Part model, mm, in its own coordinate system. A direction names the side the tool comes from. Coordinates: 2 decimals unless noted, no trailing zeros. Loops run counter-clockwise (first coordinate to the right, second up) from the corner with the lowest first, then second, coordinate; pieces in that order, holes last. Notation, with made-up numbers: (53.5, 66) -> (96.5, 66) arc R12 cw to (96.5, 89) -> close; hole circle Ø8 at (63.5, -3.5). An arc over 180 degrees is marked (long way). Use one line per item in the form item = value. Start each with the question number.
(1) Drill centre lines: L1, parallel to Z at x = 8, y = 1.5; L2, parallel to Z at x = 0.95, y = 17; L3, parallel to X at y = 23, z = 14.5. Where is each one in solid material? Low to high. Write a range as [from, to].
(2) Pin check, flat tips, straight feed: P1, Ø1.5, axis at x = 7, z = 2.5, coming from the +Y side; P2, Ø12.5, axis at y = 15, z = 15.5, coming from the +X side. Stop position of each tip, or through.
(3) Band-saw the part on A-A on z = 12.5. Give the cut face in (x, y), then the cut area to 3 significant figures.
(4) Band-saw the part on C-C on x = 24. Give the cut face in (y, z), then the cut area to 3 significant figures.
(5) 3-axis set-ups, long thin cutter, end or side, ignore diameter. For faces 5 (the flat face through (2.8, 8.7, 0)), 6 (the flat face through (17, 3, 12)): which of +Z, -Z, +X, -X, +Y, -Y reach the whole face in a straight line?
(6) Band-saw the part on D-D on z = 21. Give the cut face in (x, y), then the cut area to 3 significant figures.
(7) Band-saw the part on B-B on y = 17. Give the cut face in (x, z).
(8) Mould opens along Y. For faces 1 (the flat face through (2, 31, 12)), 2 (the cylindrical face through (1.52, 15.89, 22.01)), 3 (the cylindrical face through (28.5, 1.5, 5.1)), 4 (the cylindrical face through (1.52, 15.5, 4.07)) say: +Y half, -Y half, draft (parallel to the pull), parting line (faces both ways), or undercut.
```python
from build123d import *

# Parameters (mm, degrees)
BOSS_EXTRUDE1_DEPTH = 25
SKETCH2_R           = 1.5
SKETCH2_R_2         = 4
CUT_EXTRUDE1_DEPTH  = 49.682645779
CUT_EXTRUDE2_REACH  = 50.683
SKETCH3_R           = 2.5


with BuildPart() as part:
    # Sketch1 → Boss-Extrude1 (new body)
    with BuildSketch(Plane.XY):
        Polygon((0, 31), (0, 0), (31, 0), (31, 3), (3, 3), (3, 31), align=None)
    extrude(amount=BOSS_EXTRUDE1_DEPTH)

    # Sketch2 → Cut-Extrude1 (cut, through all)
    with BuildSketch(Plane(origin=(3, 0, 0), x_dir=(0, 0, -1), z_dir=(1, 0, 0))):
        with Locations(Location((-21, 17, 0), (0, 0, 90))):
            Circle(SKETCH2_R)
        with Locations(Location((-12.5, 17, 0), (0, 0, 90))):
            Circle(SKETCH2_R_2)
        with Locations(Location((-4, 17, 0), (0, 0, 90))):
            Circle(SKETCH2_R)
    extrude(amount=-CUT_EXTRUDE1_DEPTH, mode=Mode.SUBTRACT)

    # Sketch3 → Cut-Extrude2 (cut, up to next)
    with BuildSketch(Plane(origin=(0, 3, 0), x_dir=(1, 0, 0), z_dir=(0, 1, 0)), mode=Mode.PRIVATE) as cut_extrude2_sk1:
        with Locations(Location((8, -5, 0), (0, 0, 180))):
            Circle(SKETCH3_R)
    cut_extrude2_tool1 = extrude(cut_extrude2_sk1.sketch, amount=-CUT_EXTRUDE2_REACH, mode=Mode.PRIVATE) & part.part
    # Sketch3 → Cut-Extrude2 (cut, up to next)
    with BuildSketch(Plane(origin=(0, 3, 0), x_dir=(1, 0, 0), z_dir=(0, 1, 0)), mode=Mode.PRIVATE) as cut_extrude2_sk2:
        with Locations(Location((26, -5, 0), (0, 0, 180))):
            Circle(SKETCH3_R)
    cut_extrude2_tool2 = extrude(cut_extrude2_sk2.sketch, amount=-CUT_EXTRUDE2_REACH, mode=Mode.PRIVATE) & part.part
    # Sketch3 → Cut-Extrude2 (cut, up to next)
    with BuildSketch(Plane(origin=(0, 3, 0), x_dir=(1, 0, 0), z_dir=(0, 1, 0)), mode=Mode.PRIVATE) as cut_extrude2_sk3:
        with Locations(Location((26, -20, 0), (0, 0, 180))):
            Circle(SKETCH3_R)
    cut_extrude2_tool3 = extrude(cut_extrude2_sk3.sketch, amount=-CUT_EXTRUDE2_REACH, mode=Mode.PRIVATE) & part.part
    # Sketch3 → Cut-Extrude2 (cut, up to next)
    with BuildSketch(Plane(origin=(0, 3, 0), x_dir=(1, 0, 0), z_dir=(0, 1, 0)), mode=Mode.PRIVATE) as cut_extrude2_sk4:
        with Locations(Location((8, -20, 0), (0, 0, 180))):
            Circle(SKETCH3_R)
    cut_extrude2_tool4 = extrude(cut_extrude2_sk4.sketch, amount=-CUT_EXTRUDE2_REACH, mode=Mode.PRIVATE) & part.part
    add(cut_extrude2_tool1.solids().sort_by_distance((8, 3, 5))[0], mode=Mode.SUBTRACT)
    add(cut_extrude2_tool2.solids().sort_by_distance((26, 3, 5))[0], mode=Mode.SUBTRACT)
    add(cut_extrude2_tool3.solids().sort_by_distance((26, 3, 20))[0], mode=Mode.SUBTRACT)
    add(cut_extrude2_tool4.solids().sort_by_distance((8, 3, 20))[0], mode=Mode.SUBTRACT)


solid = part.part
```
A:
q1.L1 = [0, 2.5], [7.5, 17.5], [22.5, 25]
q1.L2 = [0, 2.5], [5.5, 8.5], [16.5, 19.5], [22.5, 25]
q1.L3 = [0, 3]
q2.P1 = 3
q2.P2 = 3
q3.outline = (0, 0) -> (31, 0) -> (31, 3) -> (3, 3) -> (3, 13) -> (0, 13) -> close; (0, 21) -> (3, 21) -> (3, 31) -> (0, 31) -> close
q3.area = 153 mm²
q4.outline = (0, 0) -> (3, 0) -> (3, 3.5) -> (0, 3.5) -> close; (0, 6.5) -> (3, 6.5) -> (3, 18.5) -> (0, 18.5) -> close; (0, 21.5) -> (3, 21.5) -> (3, 25) -> (0, 25) -> close
q4.area = 57.0 mm²
q5.face_5 = -Z, +X, -X, +Y, -Y
q5.face_6 = +Z, -Z, +X, +Y
q6.outline = (0, 0) -> (5.71, 0) -> (5.71, 3) -> (3, 3) -> (3, 15.5) -> (0, 15.5) -> close; (0, 18.5) -> (3, 18.5) -> (3, 31) -> (0, 31) -> close; (10.29, 0) -> (23.71, 0) -> (23.71, 3) -> (10.29, 3) -> close; (28.29, 0) -> (31, 0) -> (31, 3) -> (28.29, 3) -> close
q6.area = 141 mm²
q7.outline = (0, 0) -> (3, 0) -> (3, 2.5) -> (0, 2.5) -> close; (0, 5.5) -> (3, 5.5) -> (3, 8.5) -> (0, 8.5) -> close; (0, 16.5) -> (3, 16.5) -> (3, 19.5) -> (0, 19.5) -> close; (0, 22.5) -> (3, 22.5) -> (3, 25) -> (0, 25) -> close
q8.face_1 = +Y half
q8.face_2 = undercut
q8.face_3 = draft
q8.face_4 = undercut
